from build123d import *
from build123d.topology import SkipClean

# Parameters (mm, degrees)
SKETCH1_R                                         = 4.7625
BOSS_EXTRUDE1_DEPTH                               = 10.16
SKETCH3_R                                         = 16.25
BOSS_EXTRUDE2_DEPTH                               = 3.81
F_4_CLEARANCE_HOLE1_D                             = 2.9464
CUT_EXTRUDE1_START                                = -6.1595
SKETCH6_R                                         = 4.7625
SKETCH6_R_2                                       = 3.90525
CUT_EXTRUDE1_DEPTH                                = 6.1595
CUT_EXTRUDE4_DEPTH                                = 6.35
BOSS_EXTRUDE3_DEPTH                               = 2.54
CIRPATTERN1_COUNT                                 = 4
CSK_FOR_4_FLAT_HEAD_MACHINE_SCREW_100_D           = 2.9464
CSK_FOR_4_FLAT_HEAD_MACHINE_SCREW_100_CSINK_D     = 6.0177172
CSK_FOR_4_FLAT_HEAD_MACHINE_SCREW_100_CSINK_ANGLE = 100
CIRPATTERN2_COUNT                                 = 4


with BuildPart() as part:
    # Sketch1 → Boss-Extrude1 (new body)
    with BuildSketch(Plane(origin=(0, 0, 0), x_dir=(1, 0, 0), z_dir=(0, 1, 0))):
        with Locations(Location((0, 0, 0), (0, 0, 270))):
            Circle(SKETCH1_R)
    extrude(amount=BOSS_EXTRUDE1_DEPTH)

    # Sketch3 → Boss-Extrude2 (add)
    with BuildSketch(Plane.XZ):
        with Locations(Location((0, 0, 0), (0, 0, 90))):
            Circle(SKETCH3_R)
    extrude(amount=BOSS_EXTRUDE2_DEPTH)

    # #4 Clearance Hole1 (through all)
    with Locations(Plane(origin=(0, -3.81, 0), x_dir=(-1, 0, 0), z_dir=(0, -1, 0))):
        with Locations((0, 0)):
            Hole(F_4_CLEARANCE_HOLE1_D / 2)

    # Sketch6 → Cut-Extrude1 (cut)
    with BuildSketch(Plane(origin=(0, 10.16, 0), x_dir=(1, 0, 0), z_dir=(0, 1, 0)).offset(CUT_EXTRUDE1_START)):
        with Locations(Location((0, 0, 0), (0, 0, 270))):
            Circle(SKETCH6_R)
        with Locations(Location((0, 0, 0), (0, 0, 270))):
            Circle(SKETCH6_R_2, mode=Mode.SUBTRACT)
    extrude(amount=CUT_EXTRUDE1_DEPTH, mode=Mode.SUBTRACT)

    # Sketch7 → Cut-Extrude4 (cut)
    with BuildSketch(Plane.XZ.offset(3.81)):
        Polygon((-3.666174209, 0), (-1.833087105, -3.175), (1.833087105, -3.175), (3.666174209, 0), (1.833087105, 3.175), (-1.833087105, 3.175), align=None)
    extrude(amount=-CUT_EXTRUDE4_DEPTH, mode=Mode.SUBTRACT)

    # Sketch8 → Boss-Extrude3 (add)
    with BuildSketch(Plane(origin=(0, 10.16, 0), x_dir=(1, 0, 0), z_dir=(0, 1, 0))):
        with BuildLine():
            Line((-0.592971464, 1.348593001), (-1.523758258, 3.595711103))
            ThreePointArc((-1.523758258, 3.595711103), (-2.761428757, 2.761428757), (-3.595711103, 1.523758258))
            Line((-3.595711103, 1.523758258), (-1.348593001, 0.592971464))
            ThreePointArc((-1.348593001, 0.592971464), (-1.04170971, 1.04170971), (-0.592971464, 1.348593001))
        make_face()
    boss_extrude3 = extrude(amount=BOSS_EXTRUDE3_DEPTH)

    # CirPattern1: Boss-Extrude3 ×4 about axis
    with SkipClean():  # the faces are left unmerged after this step: merging them gives an invalid solid
        cirpattern1_axis = Axis((0, 0, 0), (0, 1, 0))
        for i in range(1, CIRPATTERN1_COUNT):
            add(boss_extrude3.rotate(cirpattern1_axis, i * 360 / CIRPATTERN1_COUNT))

    # CSK for #4 Flat Head Machine Screw (100)1 (through all)
    with Locations(Plane(origin=(0, 0, 0), x_dir=(1, 0, 0), z_dir=(0, 1, 0))):
        with Locations((0, 12.5)):
            csk_for_4_flat_head_machine_screw_100 = CounterSinkHole(CSK_FOR_4_FLAT_HEAD_MACHINE_SCREW_100_D / 2, CSK_FOR_4_FLAT_HEAD_MACHINE_SCREW_100_CSINK_D / 2, counter_sink_angle=CSK_FOR_4_FLAT_HEAD_MACHINE_SCREW_100_CSINK_ANGLE)

    # CirPattern2: CSK for #4 Flat Head Machine Screw (100)1 ×4 about axis
    with SkipClean():  # the faces are left unmerged after this step: merging them gives an invalid solid
        cirpattern2_axis = Axis((0, 0, 0), (0, 1, 0))
        for i in range(1, CIRPATTERN2_COUNT):
            add(csk_for_4_flat_head_machine_screw_100.rotate(cirpattern2_axis, i * 360 / CIRPATTERN2_COUNT), mode=Mode.SUBTRACT)


solid = part.part
Verification items for the finished model (mm, model axes). A direction names the side the tool comes from. Coordinates: 2 decimals unless noted, no trailing zeros. Loops run counter-clockwise (first coordinate to the right, second up) from the corner with the lowest first, then second, coordinate; pieces in that order, holes last. Notation, with made-up numbers: (46, 33) -> (55, 33) arc R22 cw to (55, 59) -> close; hole circle Ø6 at (-0.5, 83.5). An arc over 180 degrees is marked (long way). Answer as a JSON object with one key per item and string values. Group by question number.
Item 1: Sectioned sample at C-C on y = 1.75. Record the boundary of the cut face in (x, z) (1 decimal), plus the area to 3 significant figures.
Item 2: Tool access check on faces 1 (the flat face through (2.456, 11.412, -1.052)), 2 (the cylindrical face through (-2.9, 1.97, -3.78)), 3 (the flat face through (-2.456, 11.412, 1.052)). Record the directions out of +Z, -Z, +X, -X, +Y, -Y that give a thin tool (end or side, any length) a straight path to the whole face; none if there is none.
Item 3: Sectioned sample at B-B on z = 12.5. Record the boundary of the cut face in (x, y).
Item 4: Depth check by flat-ended pin: pin 1 (3.5 mm diameter, centred on x = 0, z = -12.5, fed in from +Y); pin 2 (1.1 mm diameter, centred on x = 0, y = 0.5, fed in from -Z); pin 3 (4 mm diameter, centred on x = -0.5, y = 5, fed in from +Z); pin 4 (1 mm diameter, centred on x = -10, z = -0.5, fed in from +Y). Enter the tip coordinate at first touch or a pass-through.
Item 5: Sectioned sample at D-D on x = 12.5. Record the boundary of the cut face in (y, z).
Item 6: Mould release check, pull along Z, two halves, no side actions. Record for faces 4 (the flat face through (-1.052, 11.412, -2.456)), 5 (the flat face through (2.737, -0.679, -1.61)), 6 (the cylindrical face through (-4.88, -1.88, 15.5)): +Z half, -Z half, draft (parallel to the pull), parting line (faces both ways), or undercut.
Item 7: Scan lines: probe 1 along X at (y, z) = (-2.7, 0); probe 2 along Z at (x, y) = (0, 7); probe 3 along Z at (x, y) = (-2.5, 10). Record each from-to range of solid material in increasing order.
Item 8: Sectioned sample at A-A on y = 11.5. Record the boundary of the cut face in (x, z).
Evaluation:
{
 "1": {"outline": "circle Ø9.5 at (0, 0); hole (-3.7, 0) -> (-1.8, -3.2) -> (1.8, -3.2) -> (3.7, 0) -> (1.8, 3.2) -> (-1.8, 3.2) -> close", "area": "36.3 mm²"},
 "2": {"face 1": "+X, +Y", "face 2": "+Y", "face 3": "-X, +Y"},
 "3": {"outline": "(-10.38, -3.81) -> (-1.47, -3.81) -> (-1.47, -1.29) -> (-3.01, 0) -> (-10.38, 0) -> close; (1.47, -3.81) -> (10.38, -3.81) -> (10.38, 0) -> (3.01, 0) -> (1.47, -1.29) -> close"},
 "4": {"pin 1": "stops at y = -1.06", "pin 2": "stops at z = -16.25", "pin 3": "stops at z = 4.76", "pin 4": "stops at y = 0"},
 "5": {"outline": "(-3.81, -10.38) -> (0, -10.38) -> (0, -3.01) -> (-1.29, -1.47) -> (-3.81, -1.47) -> close; (-3.81, 1.47) -> (-1.29, 1.47) -> (0, 3.01) -> (0, 10.38) -> (-3.81, 10.38) -> close"},
 "6": {"face 4": "-Z half", "face 5": "undercut", "face 6": "parting line"},
 "7": {"probe 1": "x = -16.25 to -13.97, -11.03 to -3.67, 3.67 to 11.03, 13.97 to 16.25", "probe 2": "z = -3.91 to -1.47, 1.47 to 3.91", "probe 3": "z = -3 to 3"},
 "8": {"outline": "(-3.6, -1.52) arc R3.91 ccw to (-1.52, -3.6) -> (-0.59, -1.35) arc R1.47 cw to (-1.35, -0.59) -> close; (-3.6, 1.52) -> (-1.35, 0.59) arc R1.47 cw to (-0.59, 1.35) -> (-1.52, 3.6) arc R3.91 ccw to start; (0.59, -1.35) -> (1.52, -3.6) arc R3.91 ccw to (3.6, -1.52) -> (1.35, -0.59) arc R1.47 cw to start; (0.59, 1.35) arc R1.47 cw to (1.35, 0.59) -> (3.6, 1.52) arc R3.91 ccw to (1.52, 3.6) -> close"}
}
